Could you check a few things on this drawing? It's one solid part, dimensions in mm from its lowest x, y, z. A direction names the side the tool comes from. Give positions to 0.01 mm unless a question says otherwise; leave off trailing zeros. Order: outer loops, then holes, each group sorted by start corner. A loop starts at its lowest first (then second) coordinate and runs counter-clockwise, first axis right, second up.
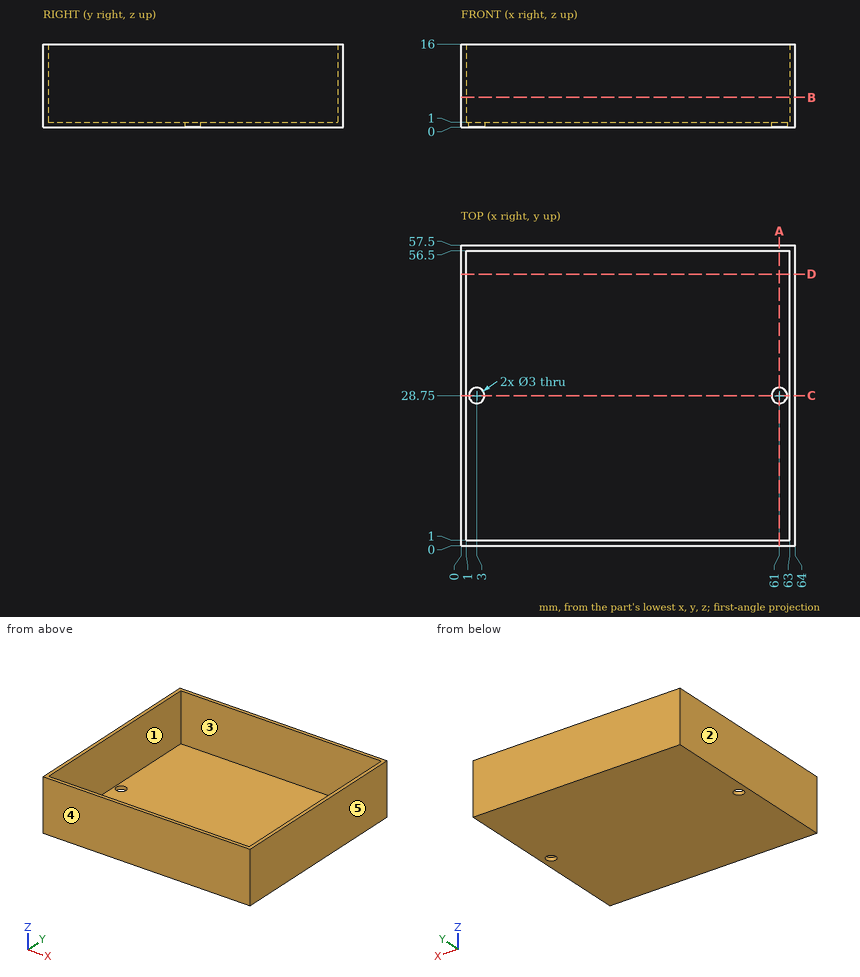
Q1. If we section it at C-C on y = 28.75: List the corners of the cut face in (x, z) for me.
Filled sheet:
outline: (0, 0) - (1.5, 0) - (1.5, 1) - (1, 1) - (1, 16) - (0, 16) - close; (4.5, 0) - (59.5, 0) - (59.5, 1) - (4.5, 1) - close; (62.5, 0) - (64, 0) - (64, 16) - (63, 16) - (63, 1) - (62.5, 1) - close
Q2. I'm going to push flat-ended pins straight in: P1, Ø6, axis at x = 14.5, y = 32.5, coming from the +Z side; P2, Ø1.8, axis at x = 3, y = 28.75, coming from the -Z side. Where does each tip first touch, or does it pass through?
Filled sheet:
P1: stops at z = 1
P2: passes through
Q3. If we section it at A-A on x = 61: List the corners of the cut face in (y, z) for me, plus the area to 3 significant figures.
Filled sheet:
outline: (0, 0) - (27.25, 0) - (27.25, 1) - (1, 1) - (1, 16) - (0, 16) - close; (30.25, 0) - (57.5, 0) - (57.5, 16) - (56.5, 16) - (56.5, 1) - (30.25, 1) - close
area: 84.5 mm2
Q4. If we section it at B-B on z = 5.75: List the corners of the cut face in (x, y) for me, plus the area to 3 significant figures.
Filled sheet:
outline: (0, 0) - (64, 0) - (64, 57.5) - (0, 57.5) - close; hole (1, 1) - (63, 1) - (63, 56.5) - (1, 56.5) - close
area: 239 mm2
Q5. For the marked faces 1 and 2, which set-ups out of +Z, -Z, +X, -X, +Y, -Y let a thin tool reach every point of the face, with its end or its side?
Filled sheet:
face 1: +Z
face 2: +Z, -Z, -X, +Y, -Y
Q6. If we section it at D-D on y = 52: List the corners of the cut face in (x, z) for me, plus the area to 3 significant figures.
Filled sheet:
outline: (0, 0) - (64, 0) - (64, 16) - (63, 16) - (63, 1) - (1, 1) - (1, 16) - (0, 16) - close
area: 94.0 mm2
Q7. Thinking about a two-plate mould opening in Y: for the marked faces 3, 4 and 5, which applies, released by +Y, released by -Y, zero draft, split by the parting line, or undercut?
Filled sheet:
face 3: undercut
face 4: released by -Y
face 5: zero draft
Q8. I need wall thicknesses on L1, parallel to X at y = 52.5, z = 8.75; L2, parallel to Y at x = 9, z = 12.25; L3, parallel to Y at x = 61, z = 0.2. Which ranges of each line are inside material? Lowest first, please.
Filled sheet:
L1: x = 0 to 1, 63 to 64
L2: y = 0 to 1, 56.5 to 57.5
L3: y = 0 to 27.25, 30.25 to 57.5
